Check sheet for the drawn part. Datum: minimum x, y, z corner. Units: mm. Coordinates: 2 decimals unless noted, no trailing zeros. Write each loop counter-clockwise with the first axis right and the second up, starting at its lowest first coordinate (ties: lowest second). Pieces come first, ordered by that corner, then holes. Notation, with made-up numbers: (34.5, 25) - (44.5, 25) arc R30 cw to (44.5, 64) - close; hole circle Ø3 at (49, 48). An arc over 180 degrees is marked (long way). Answer as CSV lines item,"result". Start each with the question number.
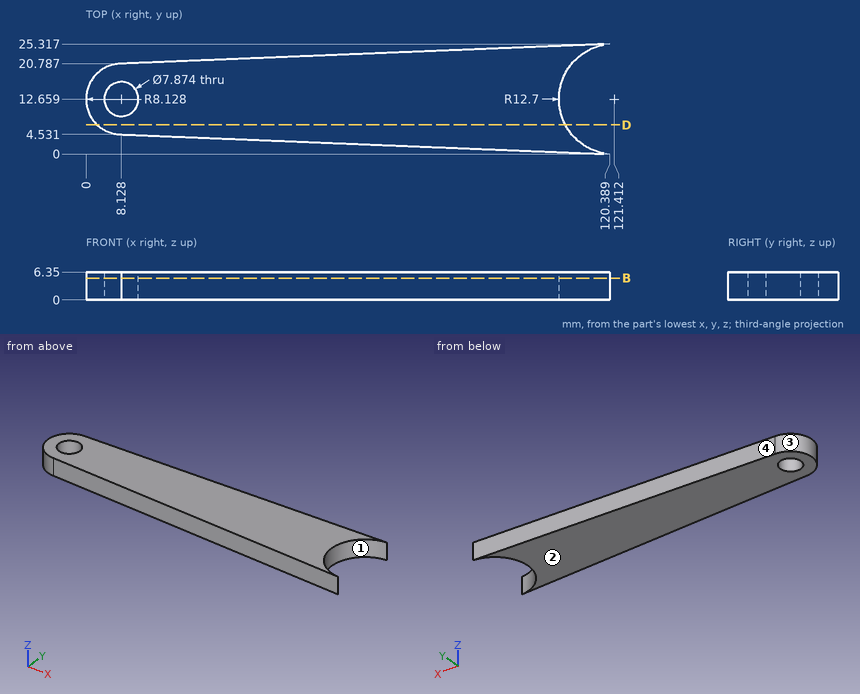
(1) Release check for a two-part mould opening along Y. For the marked faces 1, 2, 3 and 4 record: pulls with the +Y half, pulls with the -Y half, needs draft (parallel to the pull), parting line crosses it, or undercut.
(2) Cross-section at B-B on z = 5. Record the boundary of the cut face in (x, y) (1 decimal), plus the area to 3 significant figures.
(3) Material ranges on probe 1 along X at (y, z) = (13.25, 3.5) (1 decimal); probe 2 along X at (y, z) = (8, 4); probe 3 along X at (y, z) = (16.75, 5) (1 decimal), recorded low to high. Write a range as from..to.
(4) Cross-section at D-D on y = 6.75. Record the boundary of the cut face in (x, z).
(5) Go/stop test with flat-tipped pins: P1, Ø1.5, axis at x = 15, z = 5.5, coming from the -Y side; P2, Ø6.5, axis at x = 8.13, y = 12.66, coming from the +Z side; P3, Ø2, axis at x = 68, z = 1, coming from the +Y side. Record where each tip stops, or that it passes through.
Checked values:
1,face 1,"undercut"
1,face 2,"needs draft"
1,face 3,"parting line crosses it"
1,face 4,"pulls with the +Y half"
2,outline,"(8.1, 4.5) - (120.4, 0) arc R12.7 cw to (120.4, 25.3) - (8.1, 20.8) arc R8.1 ccw to start; hole circle Ø7.9 at (8.1, 12.7)"
2,area,"2,160 mm^2"
3,probe 1,"0..4.2, 12..108.7"
3,probe 2,"1.47..109.6"
3,probe 3,"1.1..109.4"
4,outline,"(2.55, 0) - (110.17, 0) - (110.17, 6.35) - (2.55, 6.35) - close"
5,P1,"y = 4.22"
5,P2,"through"
5,P3,"y = 23.24"
